from build123d import *
from build123d.topology import SkipClean

# Parameters (mm, degrees)
SKETCH1_R           = 2
BOSS_EXTRUDE1_DEPTH = 7
SKETCH2_R           = 2.05
SKETCH2_R_2         = 2
BOSS_EXTRUDE3_DEPTH = 3
SKETCH3_R           = 2.05
SKETCH3_R_2         = 2
CUT_EXTRUDE1_DEPTH  = 2.9
BOSS_EXTRUDE4_DEPTH = 4
BOSS_EXTRUDE5_START = -8
BOSS_EXTRUDE5_DEPTH = 8


with BuildPart() as part:
    # Sketch1 → Boss-Extrude1 (new body)
    with BuildSketch(Plane.XY):
        Circle(SKETCH1_R)
        with BuildLine():
            Line((0.997797575, 1.12), (0.997797575, -1.12))
            ThreePointArc((0.997797575, -1.12), (-1.5, 0), (0.997797575, 1.12))
        make_face(mode=Mode.SUBTRACT)
    extrude(amount=BOSS_EXTRUDE1_DEPTH)

    # Sketch2 → Boss-Extrude3 (add)
    with BuildSketch(Plane.XY):
        Circle(SKETCH2_R)
        Circle(SKETCH2_R_2, mode=Mode.SUBTRACT)
    extrude(amount=BOSS_EXTRUDE3_DEPTH)

    # Sketch3 → Cut-Extrude1 (cut)
    with BuildSketch(Plane.XY):
        Circle(SKETCH3_R)
        Circle(SKETCH3_R_2, mode=Mode.SUBTRACT)
    extrude(amount=CUT_EXTRUDE1_DEPTH, mode=Mode.SUBTRACT)

    # Sketch4 → Boss-Extrude4 (add)
    with SkipClean():  # the faces are left unmerged after this step: merging them gives an invalid solid
        with BuildSketch(Plane.XY.offset(7)):
            with BuildLine():
                Line((1.854049622, 0.75), (2.125, 0.75))
                Line((2.125, 0.75), (2.125, -0.75))
                Line((2.125, -0.75), (1.854049622, -0.75))
                ThreePointArc((1.854049622, -0.75), (0, -2), (-1.854049622, -0.75))
                Line((-1.854049622, -0.75), (-2.125, -0.75))
                Line((-2.125, -0.75), (-2.125, 0.75))
                Line((-2.125, 0.75), (-1.854049622, 0.75))
                ThreePointArc((-1.854049622, 0.75), (0, 2), (1.854049622, 0.75))
            make_face()
        extrude(amount=BOSS_EXTRUDE4_DEPTH)

    # Sketch8 → Boss-Extrude5 (add)
    with BuildSketch(Plane.XY.offset(11).offset(BOSS_EXTRUDE5_START)):
        with BuildLine():
            Line((1.854049622, -0.75), (2.125, -0.75))
            Line((2.125, -0.75), (2.125, 0.75))
            Line((2.125, 0.75), (1.854049622, 0.75))
            ThreePointArc((1.854049622, 0.75), (2, 0), (1.854049622, -0.75))
        make_face()
        with BuildLine():
            Line((-2.125, -0.75), (-1.854049622, -0.75))
            ThreePointArc((-1.854049622, -0.75), (-2, 0), (-1.854049622, 0.75))
            Line((-1.854049622, 0.75), (-2.125, 0.75))
            Line((-2.125, 0.75), (-2.125, -0.75))
        make_face()
    extrude(amount=BOSS_EXTRUDE5_DEPTH)


solid = part.part
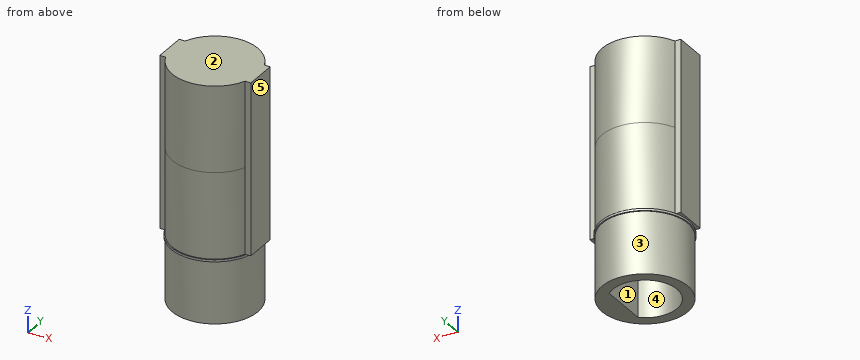
Read the model definition and answer for the solid it produces. Units are mm, in the model's axes. Face numbers are marked on the shaded views. A direction names the side the tool comes from. Round coordinates to 2 decimals unless told otherwise and drop trailing zeros. Loops run counter-clockwise (first coordinate to the right, second up) from the corner with the lowest first, then second, coordinate; pieces in that order, holes last.
Q1. Consider probe 1 along Y at (x, z) = (0.1, 2.25); probe 2 along Z at (x, y) = (0.35, 0.9); probe 3 along Y at (x, z) = (2, 4). Determine where each line is inside the solid, lowest interval first.
Q2. This flat-tipped pin is pushed along its axis until it touches: pin 1 (2 mm diameter, centred on x = 1.5, z = 7, fed in from +Y). Where does it stop, or does it pass through?
Q3. Section B-B on x = 0 is taken. Write down the section's boundary in (y, z).
Q4. Section A-A on z = 4.75 is taken. Write down the section's boundary in (x, y) (3 decimals).
Q5. Section C-C on y = 0 is taken. Write down the section's boundary in (x, z) (3 decimals).
Q6. Which of the six approach directions +Z, -Z, +X, -X, +Y, -Y give full straight-line access (tool end or side, diameter ignored) to the marked faces 4 and 5?
Q7. Determine the mould class of the marked faces 1, 2 and 3 for opening direction X: released by +X, released by -X, zero draft, split by the parting line, or undercut.
Q8. Section D-D on z = 2.5 is taken. Write down the section's boundary in (x, y).
Output:
1. probe 1: y = -2 to -1.5, 1.5 to 2
1. probe 2: z = 7 to 11
1. probe 3: y = -0.75 to 0.75
2. pin 1: stops at y = 1.94
3. outline: (-2.05, 2.9) - (-2, 2.9) - (-2, 0) - (-1.5, 0) - (-1.5, 7) - (1.5, 7) - (1.5, 0) - (2, 0) - (2, 2.9) - (2.05, 2.9) - (2.05, 3) - (2, 3) - (2, 11) - (-2, 11) - (-2, 3) - (-2.05, 3) - close
4. outline: (-2.125, -0.75) - (-1.854, -0.75) arc R2 ccw to (1.854, -0.75) - (2.125, -0.75) - (2.125, 0.75) - (1.854, 0.75) arc R2 ccw to (-1.854, 0.75) - (-2.125, 0.75) - close; hole (0.998, -1.12) - (0.998, 1.12) arc R1.5 ccw (long way) to start
5. outline: (-2.125, 3) - (-2.05, 3) - (-2.05, 2.9) - (-2, 2.9) - (-2, 0) - (-1.5, 0) - (-1.5, 7) - (0.998, 7) - (0.998, 0) - (2, 0) - (2, 2.9) - (2.05, 2.9) - (2.05, 3) - (2.125, 3) - (2.125, 11) - (-2.125, 11) - close
6. face 4: -Z
6. face 5: +Z, -Z, +X, +Y, -Y
7. face 1: undercut
7. face 2: zero draft
7. face 3: split by the parting line
8. outline: circle Ø4 at (0, 0); hole (1, -1.12) - (1, 1.12) arc R1.5 ccw (long way) to start
